```python
from build123d import *

# Parameters (mm, degrees)
ODGI_CIE_BAZOWE1_DEPTH      = 30
OTW_R_POD_RUB_M51_D         = 5.5
OTW_R_POD_RUB_M51_DEPTH     = 14
OTW_R_POD_RUB_M51_TIP       = 1.652366702
DODANIE_WYCI_GNI_CIE1_DEPTH = 2
DODANIE_WYCI_GNI_CIE2_DEPTH = 2
WYTNIJ_WYCI_GNI_CIE1_DEPTH  = 10
WYTNIJ_WYCI_GNI_CIE3_DEPTH  = 10


# Sheet-metal steps are written as plain solids
with BuildPart() as part:
    # Szkic1 → Odgięcie bazowe1 (new body)
    with BuildSketch(Plane.XY):
        with BuildLine():
            Line((0, 405.16), (73.22194051, 280.801279174))
            ThreePointArc((73.22194051, 280.801279174), (73.876553772, 279.249103741), (74.1, 277.579421472))
            Line((74.1, 277.579421472), (74.1, 127.580578528))
            ThreePointArc((74.1, 127.580578528), (73.876553772, 125.910896259), (73.22194051, 124.358720826))
            Line((73.22194051, 124.358720826), (0, 0))
            Line((0, 0), (1.72344583, -1.014758331))
            Line((1.72344583, -1.014758331), (74.94538634, 123.343962495))
            ThreePointArc((74.94538634, 123.343962495), (75.806177007, 125.38501208), (76.1, 127.580578528))
            Line((76.1, 127.580578528), (76.1, 277.579421472))
            ThreePointArc((76.1, 277.579421472), (75.806177007, 279.77498792), (74.94538634, 281.816037505))
            Line((74.94538634, 281.816037505), (1.72344583, 406.174758331))
            Line((1.72344583, 406.174758331), (0, 405.16))
        make_face()
    extrude(amount=ODGI_CIE_BAZOWE1_DEPTH)

    # Otwór pod śrubę M51
    with Locations(Plane(origin=(76.1, 0, 0), x_dir=(0, 0, -1), z_dir=(1, 0, 0))):
        with Locations((-15, 157.580578528), (-15, 247.579421472)):
            Hole(OTW_R_POD_RUB_M51_D / 2, depth=OTW_R_POD_RUB_M51_DEPTH)
            with Locations((0, 0, -(OTW_R_POD_RUB_M51_DEPTH + OTW_R_POD_RUB_M51_TIP / 2))):  # 118° drill point
                Cone(0, OTW_R_POD_RUB_M51_D / 2, OTW_R_POD_RUB_M51_TIP, mode=Mode.SUBTRACT)

    # Szkic10 → Dodanie-wyciągnięcie1 (add)
    with BuildSketch(Plane(origin=(178.867603803, 105.316562907, 0), x_dir=(0, 0, -1), z_dir=(0.8617229149967045, 0.5073791656833994, 0))):
        Polygon((-30, 349.13565624), (-0.000160653, 354.682794047), (0, 349.13565624), align=None)
    extrude(amount=-DODANIE_WYCI_GNI_CIE1_DEPTH)

    # Szkic11 → Dodanie-wyciągnięcie2 (add)
    with BuildSketch(Plane(origin=(1.72344583, -1.014758331, 0), x_dir=(0, 0, -1), z_dir=(0.8617229149967046, -0.507379165683399, 0))):
        Polygon((-30, 0), (0.008092813, -8.531045483), (0, 0), align=None)
    extrude(amount=-DODANIE_WYCI_GNI_CIE2_DEPTH)

    # Szkic13 → Wytnij-wyciągnięcie1 (cut)
    with BuildSketch(Plane(origin=(0, 0, 0), x_dir=(0, 0, 1), z_dir=(-0.8617229149967046, 0.5073791656833994, 0))):
        with BuildLine():
            Line((7.495953593, 10.734477259), (7.495953593, 50.734477259))
            ThreePointArc((7.495953593, 50.734477259), (14.995953593, 58.234477259), (22.495953593, 50.734477259))
            Line((22.495953593, 50.734477259), (22.495953593, 10.734477259))
            ThreePointArc((22.495953593, 10.734477259), (14.995953593, 3.234477259), (7.495953593, 10.734477259))
        make_face()
        with BuildLine():
            Line((7.495953593, 83.234477259), (7.495953593, 123.234477259))
            ThreePointArc((7.495953593, 123.234477259), (14.995953593, 130.734477259), (22.495953593, 123.234477259))
            Line((22.495953593, 123.234477259), (22.495953593, 83.234477259))
            ThreePointArc((22.495953593, 83.234477259), (14.995953593, 75.734477259), (7.495953593, 83.234477259))
        make_face()
    extrude(amount=-WYTNIJ_WYCI_GNI_CIE1_DEPTH, mode=Mode.SUBTRACT)

    # Szkic12 → Wytnij-wyciągnięcie3 (cut)
    with BuildSketch(Plane(origin=(177.144157973, 104.301804576, 0), x_dir=(0, 0, 1), z_dir=(-0.8617229149967045, -0.5073791656833994, 0))):
        with BuildLine():
            Line((22.500080327, 335.4184445), (22.500080327, 295.4184445))
            ThreePointArc((22.500080327, 295.4184445), (15.000080327, 287.9184445), (7.500080327, 295.4184445))
            Line((7.500080327, 295.4184445), (7.500080327, 335.4184445))
            ThreePointArc((7.500080327, 335.4184445), (15.000080327, 342.9184445), (22.500080327, 335.4184445))
        make_face()
        with BuildLine():
            Line((22.500080327, 262.9184445), (22.500080327, 222.9184445))
            ThreePointArc((22.500080327, 222.9184445), (15.000080327, 215.4184445), (7.500080327, 222.9184445))
            Line((7.500080327, 222.9184445), (7.500080327, 262.9184445))
            ThreePointArc((7.500080327, 262.9184445), (15.000080327, 270.4184445), (22.500080327, 262.9184445))
        make_face()
    extrude(amount=-WYTNIJ_WYCI_GNI_CIE3_DEPTH, mode=Mode.SUBTRACT)


solid = part.part
```
Geometry check sheet. Reference: the model listing, model coordinates, mm. A direction names the side the tool comes from. Coordinates: 2 decimals unless noted, no trailing zeros. Loops run counter-clockwise (first coordinate to the right, second up) from the corner with the lowest first, then second, coordinate; pieces in that order, holes last. Notation, with made-up numbers: (16, 21) - (23, 21) arc R21 cw to (23, 34) - close; hole circle Ø7 at (36, 24.25). An arc over 180 degrees is marked (long way). One line per item, written item: value. Start each with the question number.
(1) Mould release check, pull along Y, two halves, no side actions. Record for faces 1 (the cylindrical face through (39.28, 64.76, 15.16)), 2 (the cylindrical face through (67.181, 112.155, 14.831)), 3 (the flat face through (76.1, 202, 15)): released by +Y, released by -Y, zero draft, split by the parting line, or undercut.
(2) Depth check by flat-ended pin: P1, Ø5, axis at x = 59, z = 23.5, coming from the -Y side; P2, Ø5, axis at x = 0.5, y = 407, coming from the -Z side; P3, Ø5, axis at y = 261, z = 17.5, coming from the -X side; P4, Ø6.5, axis at x = 19, y = 369, coming from the +Z side. Enter the tip coordinate at first touch or a pass-through.
(3) Material ranges on line 1 (Y direction, x = 74.65, z = 15); line 2 (Y direction, x = 75.2, z = 15); line 3 (X direction, y = 206, z = 15), recorded low to high. Write a range as [from, to].
(4) Cross-section at A-A on y = 19.5. Enter the section's corners in (x, z).
(5) Tool access check on faces 4 (the cylindrical face through (31.91, 352.91, 15.17)), 5 (the cylindrical face through (2.49, 2.29, 15.16)). Record the directions out of +Z, -Z, +X, -X, +Y, -Y that give a thin tool (end or side, any length) a straight path to the whole face; none if there is none.
Results below:
1. face 1: undercut
1. face 2: released by -Y
1. face 3: zero draft
2. P1: stops at y = 92.02
2. P2: stops at z = 0
2. P3: stops at x = 74.1
2. P4: stops at z = 30
3. line 1: y = [122.84, 154.83], [160.33, 244.83], [250.33, 282.32]
3. line 2: y = [123.81, 154.83], [160.33, 244.83], [250.33, 281.35]
3. line 3: x = [74.1, 76.1]
4. outline: (11.48, 0) - (13.8, 0) - (13.8, 7.5) - (11.48, 7.5) - close; (11.48, 22.5) - (13.8, 22.5) - (13.8, 30) - (11.48, 30) - close
5. face 4: -X, +Y
5. face 5: +X
